Verification items for the finished model (mm, model axes). Face numbers are marked on the shaded views. Give positions to 0.01 mm unless a question says otherwise; leave off trailing zeros. Order: outer loops, then holes, each group sorted by start corner. A loop starts at its lowest first (then second) coordinate and runs counter-clockwise, first axis right, second up. Notation, with made-up numbers: (-37.5, -15.75) -> (-31.5, -15.75) arc R21 ccw to (-31.5, -0.75) -> close; hole circle Ø5 at (63, 38.5). An arc over 180 degrees is marked (long way). Return JSON: item names as keys, results as strings. Group by question number.
(1) Cross-section at B-B on x = -75. Enter the section's corners in (y, z), then the cut area to 3 significant figures.
(2) Release check for a two-part mould opening along Y. For the marked faces 1, 2 and 3 record: pulls with the +Y half, pulls with the -Y half, needs draft (parallel to the pull), parting line crosses it, or undercut.
(3) Cross-section at A-A on z = -10. Enter the section's corners in (x, y).
(4) Depth check by flat-ended pin: pin 1 Ø6 at (x, y) = (60.5, 11.5) entering from -Z; pin 2 Ø5.5 at (x, z) = (-75, -30) entering from +Y. Enter the tip coordinate at first touch or a pass-through.
(5) Thickness scan on line 1 along Z through (x, y) = (75, 0.85); line 2 along Y through (x, z) = (-2.5, -11); line 3 along Z through (x, y) = (-17.5, 17). Record the ranges inside material, lowest first.
(6) Cross-section at C-C on y = 10. Enter the section's corners in (x, z), then the cut area to 3 significant figures.
(7) Cross-section at D-D on x = 41. Enter the section's corners in (y, z).
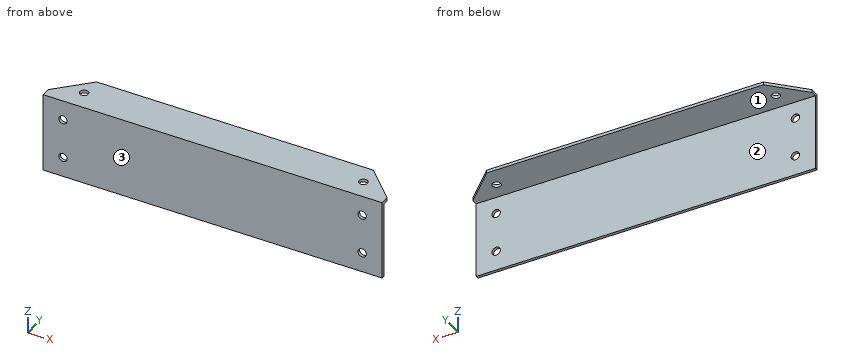
from build123d import *

# Parameters (mm, degrees)
PAD_DEPTH     = 85
SKETCH002_R   = 2.1
HOLE_DEPTH    = 20.001
SKETCH003_R   = 2.1
HOLE001_DEPTH = 40.001
POCKET_DEPTH  = 391.568917


with BuildPart() as part:
    # Sketch → Pad (new body, symmetric)
    with BuildSketch(Plane.YZ):
        Polygon((0, -40), (0, 0), (20, 0), (20, -1.5), (1.5, -1.5), (1.5, -40), align=None)
    extrude(amount=PAD_DEPTH, both=True)

    # Sketch002 → Hole (cut, through all)
    with BuildSketch(Plane.XZ):
        with Locations((-75, -30)):
            Circle(SKETCH002_R)
        with Locations((75, -30)):
            Circle(SKETCH002_R)
        with Locations((-75, -10)):
            Circle(SKETCH002_R)
        with Locations((75, -10)):
            Circle(SKETCH002_R)
    extrude(amount=-HOLE_DEPTH, mode=Mode.SUBTRACT)

    # Sketch003 → Hole001 (cut, through all)
    with BuildSketch(Plane.XY):
        with Locations((-70, 10)):
            Circle(SKETCH003_R)
        with Locations((70, 10)):
            Circle(SKETCH003_R)
    extrude(amount=-HOLE001_DEPTH, mode=Mode.SUBTRACT)

    # Sketch004 → Pocket (cut, through all)
    with BuildSketch(Plane.XY):
        Polygon((-85, 4.377634), (-85, 50), (-39.377634, 50), align=None)
    pocket = extrude(amount=-POCKET_DEPTH, mode=Mode.SUBTRACT)

    # Mirrored: Pocket across YZ
    add(pocket.mirror(Plane.YZ), mode=Mode.SUBTRACT)


solid = part.part
Verdict:
{
 "1": {"outline": "(0, -40) -> (1.5, -40) -> (1.5, -32.1) -> (0, -32.1) -> close; (0, -27.9) -> (1.5, -27.9) -> (1.5, -12.1) -> (0, -12.1) -> close; (0, -7.9) -> (1.5, -7.9) -> (1.5, -1.5) -> (14.38, -1.5) -> (14.38, 0) -> (0, 0) -> close", "area": "66.7 mm²"},
 "2": {"face 1": "needs draft", "face 2": "pulls with the +Y half", "face 3": "pulls with the -Y half"},
 "3": {"outline": "(-85, 0) -> (-77.1, 0) -> (-77.1, 1.5) -> (-85, 1.5) -> close; (-72.9, 0) -> (72.9, 0) -> (72.9, 1.5) -> (-72.9, 1.5) -> close; (77.1, 0) -> (85, 0) -> (85, 1.5) -> (77.1, 1.5) -> close"},
 "4": {"pin 1": "z = -1.5", "pin 2": "y = 1.5"},
 "5": {"line 1": "-40 to -32.1, -27.9 to -12.1, -7.9 to 0", "line 2": "0 to 1.5", "line 3": "-1.5 to 0"},
 "6": {"outline": "(-79.38, -1.5) -> (-72.1, -1.5) -> (-72.1, 0) -> (-79.38, 0) -> close; (-67.9, -1.5) -> (67.9, -1.5) -> (67.9, 0) -> (-67.9, 0) -> close; (72.1, -1.5) -> (79.38, -1.5) -> (79.38, 0) -> (72.1, 0) -> close", "area": "226 mm²"},
 "7": {"outline": "(0, -40) -> (1.5, -40) -> (1.5, -1.5) -> (20, -1.5) -> (20, 0) -> (0, 0) -> close"}
}
